from build123d import *

# Parameters (mm, degrees)
SKETCH1_R           = 25
SKETCH1_R_2         = 9.5
BOSS_EXTRUDE1_DEPTH = 15
SKETCH2_R           = 25
SKETCH2_R_2         = 14
BOSS_EXTRUDE2_DEPTH = 4
CUT_EXTRUDE1_DEPTH  = 43.178193418
CIRPATTERN1_COUNT   = 9


with BuildPart() as part:
    # Sketch1 → Boss-Extrude1 (new body)
    with BuildSketch(Plane(origin=(0, 0, 0), x_dir=(1, 0, 0), z_dir=(0, 1, 0))):
        with Locations(Location((0, 0, 0), (0, 0, 270))):
            Circle(SKETCH1_R)
        with Locations(Location((0, 0, 0), (0, 0, 270))):
            Circle(SKETCH1_R_2, mode=Mode.SUBTRACT)
    extrude(amount=BOSS_EXTRUDE1_DEPTH)

    # Sketch2 → Boss-Extrude2 (add)
    with BuildSketch(Plane(origin=(0, 15, 0), x_dir=(1, 0, 0), z_dir=(0, 1, 0))):
        with Locations(Location((0, 0, 0), (0, 0, 270))):
            Circle(SKETCH2_R)
        with Locations(Location((0, 0, 0), (0, 0, 270))):
            Circle(SKETCH2_R_2, mode=Mode.SUBTRACT)
    boss_extrude2 = extrude(amount=BOSS_EXTRUDE2_DEPTH)

    # Mirror1: Boss-Extrude2 across plane
    add(boss_extrude2.mirror(Plane.ZX.offset(7.5)))

    # Sketch6 → Cut-Extrude1 (cut, through all)
    with BuildSketch(Plane.XZ.offset(4)):
        with BuildLine():
            Line((-3.479327524, 24.756701719), (-2.644288918, 18.815093306))
            ThreePointArc((-2.644288918, 18.815093306), (-1.325373001, 18.953716955), (0, 19))
            Line((0, 19), (0, 25))
            ThreePointArc((0, 25), (-1.743911844, 24.939101256), (-3.479327524, 24.756701719))
        make_face()
    cut_extrude1 = extrude(amount=-CUT_EXTRUDE1_DEPTH, mode=Mode.SUBTRACT)

    # CirPattern1: Cut-Extrude1 ×9 about axis
    cirpattern1_axis = Axis((0, 0, 0), (0, 1, 0))
    for i in range(1, CIRPATTERN1_COUNT):
        add(cut_extrude1.rotate(cirpattern1_axis, i * 360 / CIRPATTERN1_COUNT), mode=Mode.SUBTRACT)


solid = part.part
Could you check a few things on this model? Use its own coordinates, in mm. A direction names the side the tool comes from. Give positions to 0.01 mm unless a question says otherwise; leave off trailing zeros. Order: outer loops, then holes, each group sorted by start corner. A loop starts at its lowest first (then second) coordinate and runs counter-clockwise, first axis right, second up. Notation, with made-up numbers: (-4.75, 10.25) - (-0.75, 10.25) arc R9 cw to (-0.75, 25.25) - close; hole circle Ø5 at (-13, 28). An arc over 180 degrees is marked (long way). One line per item, written item: value. Start each with the question number.
1. Imagine slicing it at B-B on x = 20.5. List the corners of the cut face in (y, z) for me, plus the area to 3 significant figures.
2. Imagine slicing it at D-D on z = 10.5. List the corners of the cut face in (x, y) for me, plus the area to 3 significant figures.
3. For P1, Ø10, axis at x = 0.5, z = 6.5, coming from the -Y side; P2, Ø1.5, axis at y = 10, z = -10, coming from the +X side; P3, Ø3, axis at x = -17, y = 3, coming from the -Z side; P4, Ø22.5, axis at x = -4, z = 2, coming from the +Y side, each with a flat end and sliding along its axis, tell me the tip position at first contact or that it passes through.
4. Imagine slicing it at C-C on x = -11. List the corners of the cut face in (y, z) for me.
5. Thinking about a two-plate mould opening in Z: for faces 1 (the face through (-11, -4, 11)), 2 (the face through (-17.37, 7.34, -13.57)), 3 (the face through (-13.67, 16.97, -3.03)), 4 (the face through (-1.344, 7.339, 18.952)), which applies, +Z half, -Z half, draft (parallel to the pull), parting line (faces both ways), or undercut?
6. Imagine slicing it at A-A on z = 0. List the corners of the cut face in (x, y) for me, plus the area to 3 significant figures.
7. For faces 5 (the face through (10.348, 7.339, -19.462)), 6 (the face through (19.02, 7.34, -10.98)), 7 (the face through (-3.07, 7.34, 21.83)), 8 (the face through (-13.212, 7.339, 13.655)), 9 (the face through (-21.624, 7.339, 3.813)), which set-ups out of +Z, -Z, +X, -X, +Y, -Y let a thin tool reach every point of the face, with its end or its side?
8. If I drill on probe 1 along X at (y, z) = (15.8, 0); probe 2 along Z at (x, y) = (-5.5, 11.5); probe 3 along X at (y, z) = (7.5, 0), over which ranges is the centre line in solid material (lowest first)?
Values:
1. outline: (-4, -14.31) - (19, -14.31) - (19, -11.84) - (-4, -11.84) - close; (-4, -8.28) - (19, -8.28) - (19, 3.61) - (-4, 3.61) - close; (-4, 6.66) - (19, 6.66) - (19, 14.31) - (-4, 14.31) - close
1. area: 506 mm²
2. outline: (-22.69, -4) - (-9.26, -4) - (-9.26, 0) - (9.26, 0) - (9.26, -4) - (22.69, -4) - (22.69, 19) - (9.26, 19) - (9.26, 15) - (-9.26, 15) - (-9.26, 19) - (-22.69, 19) - close
2. area: 895 mm²
3. P1: y = 0
3. P2: x = 23.23
3. P3: z = -19.62
3. P4: y = 19
4. outline: (-4, -22.45) - (19, -22.45) - (19, -8.66) - (15, -8.66) - (15, 8.66) - (19, 8.66) - (19, 22.45) - (-4, 22.45) - (-4, 8.66) - (0, 8.66) - (0, -8.66) - (-4, -8.66) - close
5. face 1: draft
5. face 2: undercut
5. face 3: undercut
5. face 4: +Z half
6. outline: (-25, -4) - (-14, -4) - (-14, 0) - (-9.5, 0) - (-9.5, 15) - (-14, 15) - (-14, 19) - (-25, 19) - close; (9.5, 0) - (14, 0) - (14, -4) - (25, -4) - (25, 19) - (14, 19) - (14, 15) - (9.5, 15) - close
6. area: 641 mm²
7. face 5: -Z, +Y, -Y
7. face 6: +X, +Y, -Y
7. face 7: +Z, +Y, -Y
7. face 8: +Y, -Y
7. face 9: -X, +Y, -Y
8. probe 1: -25 to -14, 14 to 25
8. probe 2: -18.19 to -7.75, 7.75 to 24.39
8. probe 3: -25 to -9.5, 9.5 to 25
